Read the model definition and answer for the solid it produces. Units are mm, in the model's axes. Give positions to 0.01 mm unless a question says otherwise; leave off trailing zeros. Write each loop counter-clockwise with the first axis right and the second up, starting at its lowest first coordinate (ties: lowest second). Pieces come first, ordered by that corner, then holes.
```python
from build123d import *

# Parameters (mm, degrees)
BOSS_EXTRUDE1_DEPTH = 6.35
CUT_EXTRUDE1_DEPTH  = 6.35


with BuildPart() as part:
    # Sketch1 → Boss-Extrude1 (new body)
    with BuildSketch(Plane(origin=(0, 0, 0), x_dir=(0, 0, -1), z_dir=(1, 0, 0))):
        with BuildLine():
            Line((0, 250), (521.678128656, 314.05401996))
            ThreePointArc((521.678128656, 314.05401996), (539.766779046, 327.550652044), (546.65, 349.044363214))
            Line((546.65, 349.044363214), (546.65, 425.274363214))
            Line((546.65, 425.274363214), (613, 425.274363214))
            Line((613, 425.274363214), (613, 398.924363214))
            Line((613, 398.924363214), (606.65, 398.924363214))
            Line((606.65, 398.924363214), (606.65, 348.924363214))
            Line((606.65, 348.924363214), (613, 348.924363214))
            Line((613, 348.924363214), (613, 328.939575476))
            Line((613, 328.939575476), (606.65, 328.939575476))
            Line((606.65, 328.939575476), (606.65, 278.939575476))
            Line((606.65, 278.939575476), (613, 278.939575476))
            Line((613, 278.939575476), (613, 258.954787738))
            Line((613, 258.954787738), (606.65, 258.954787738))
            Line((606.65, 258.954787738), (606.65, 208.954787738))
            Line((606.65, 208.954787738), (613, 208.954787738))
            Line((613, 208.954787738), (613, 188.97))
            Line((613, 188.97), (606.65, 188.97))
            Line((606.65, 188.97), (606.65, 138.97))
            Line((606.65, 138.97), (613, 138.97))
            Line((613, 138.97), (613, 0))
            Line((613, 0), (0, 0))
            Line((0, 0), (0, 50))
            Line((0, 50), (-12.7, 50))
            Line((-12.7, 50), (-12.7, 100))
            Line((-12.7, 100), (0, 100))
            Line((0, 100), (0, 160))
            Line((0, 160), (-12.7, 160))
            Line((-12.7, 160), (-12.7, 210))
            Line((-12.7, 210), (0, 210))
            Line((0, 210), (0, 250))
        make_face()
    extrude(amount=BOSS_EXTRUDE1_DEPTH)

    # Sketch2 → Cut-Extrude1 (cut)
    with BuildSketch(Plane(origin=(6.35, 0, 0), x_dir=(0, 0, -1), z_dir=(1, 0, 0))):
        Polygon((61.537861402, 231.965149724), (62.311731732, 225.662481662), (111.939039314, 231.755948832), (111.165168984, 238.058616895), align=None)
        Polygon((220.345245664, 251.464244669), (170.717938082, 245.370777499), (171.491808413, 239.068109436), (221.119115995, 245.161576606), align=None)
        Polygon((329.525322345, 264.869872444), (279.898014763, 258.776405274), (280.671885093, 252.473737211), (330.299192676, 258.567204381), align=None)
        Polygon((438.705399025, 278.275500218), (389.078091443, 272.182033048), (389.851961774, 265.879364985), (439.479269356, 271.972832155), align=None)
        Polygon((547.885475706, 291.681127993), (498.258168124, 285.587660823), (499.032038455, 279.28499276), (548.659346037, 285.37845993), align=None)
    extrude(amount=-CUT_EXTRUDE1_DEPTH, mode=Mode.SUBTRACT)


solid = part.part
```
Item 1: Each of these flat-tipped pins is pushed along its axis until it touches: pin 1 Ø3 at (x, y) = (3.5, 242) entering from -Z; pin 2 Ø1.9 at (x, y) = (2, 221) entering from +Z; pin 3 Ø3 at (x, z) = (4.5, 6) entering from +Y. Where does it stop, or does it pass through?
Result set:
pin 1: stops at z = -606.65
pin 2: stops at z = 0
pin 3: stops at y = 210
Item 2: Section A-A (z = -72.5) is taken. Write down the section's boundary in (x, y), and give its area (3 significant figures).
Result set:
outline: (0, 0) - (6.35, 0) - (6.35, 226.91) - (0, 226.91) - close; (0, 233.31) - (6.35, 233.31) - (6.35, 258.9) - (0, 258.9) - close
area: 1,600 mm2
Item 3: Section B-B (y = 381) is taken. Write down the section's boundary in (x, z), and give its area (3 significant figures).
Result set:
outline: (0, -606.65) - (6.35, -606.65) - (6.35, -546.65) - (0, -546.65) - close
area: 381 mm2
Item 4: Section C-C (x = 5) is taken. Give the number of separate pieces and of enclosed holes in the cut face, and give its area (3 significant figures).
Result set:
separate pieces: 1
enclosed holes: 5
area: 182,000 mm2
Item 5: Section D-D (z = -431) is taken. Write down the section's boundary in (x, y), and give its area (3 significant figures).
Result set:
outline: (0, 0) - (6.35, 0) - (6.35, 270.93) - (0, 270.93) - close; (0, 277.33) - (6.35, 277.33) - (6.35, 302.92) - (0, 302.92) - close
area: 1,880 mm2
Item 6: Find the intervals of material crossed by line 1 along Z through (x, y) = (2.75, 221); line 2 along Z through (x, y) = (5.25, 359); line 3 along Y through (x, z) = (2.5, -20), in increasing order.
Result set:
line 1: z = -606.65 to 0
line 2: z = -606.65 to -546.65
line 3: y = 0 to 252.46
